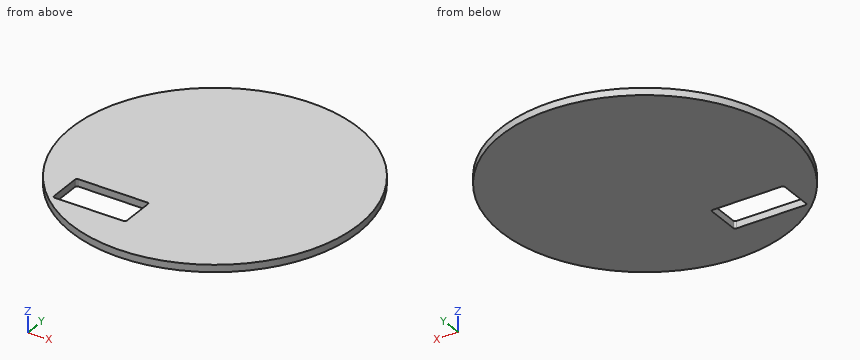
Autodesk Inventor part; units mm, degrees
ref_plane "YZ Plane" through (0, 0, 0) normal (1, 0, 0) x (0, 1, 0)
ref_plane "XZ Plane" through (0, 0, 0) normal (0, 1, 0) x (-1, 0, 0)
ref_plane "XY Plane" through (0, 0, 0) normal (0, 0, 1) x (1, 0, 0)
sketch "Эскиз1" plane through (0, 0, 0) normal (0, 0, 1) x (1, 0, 0)
  circle A0 centre (0, 0) radius 80
  line L0 (-52.7593, -38.063) -> (-52.778, -56.063)
  line L1 (-14.2583, -37.1029) -> (-50.7583, -37.0651)
  line L2 (-12.278, -56.105) -> (-12.2594, -38.105)
  line L3 (-50.779, -57.0651) -> (-14.279, -57.1029)
  line L4 (-51.7583, -37.063) -> (-13.279, -37.063)
  line L5 (-12.279, -38.063) -> (-12.279, -56.105)
  line L6 (-13.279, -57.105) -> (-51.7583, -57.105)
  line L7 (-52.7583, -56.105) -> (-52.7583, -38.063)
  arc A1 (-52.7583, -56.105) -> (-51.7583, -57.105) centre (-51.7583, -56.105) ccw
  arc A2 (-51.7583, -37.063) -> (-52.7583, -38.063) centre (-51.7583, -38.063) ccw
  arc A3 (-13.279, -57.105) -> (-12.279, -56.105) centre (-13.279, -56.105) ccw
  arc A4 (-12.279, -38.063) -> (-13.279, -37.063) centre (-13.279, -38.063) ccw
  point P0 (-52.7583, -37.063)
  dimension "d2" = 160
  dimension "d3" = 1
extrude "Выдавливание1" add sketch "Эскиз1" against normal blind 4
properties part number "нижний эллипс головы"
Build history of the part. All positions in model axes, mm. Round coordinates to 2 decimals unless told otherwise and drop trailing zeros. Loops run counter-clockwise (first coordinate to the right, second up) from the corner with the lowest first, then second, coordinate; pieces in that order, holes last.
Item 1: Saw through at D-D (x = 48). List the corners of the cut face in (y, z), then the cut area to 3 significant figures.
Item 2: Pin check, flat tips, straight feed: P1, Ø2, axis at x = -33.5, z = -2.5, coming from the +Y side; P2, Ø2, axis at y = -51, z = -1.5, coming from the +X side; P3, Ø2, axis at y = -43, z = -1, coming from the -X side. Stop position of each tip, or through.
Item 3: Saw through at A-A (z = -0.85). List the corners of the cut face in (x, y) (3 decimals).
Item 4: Saw through at C-C (y = 14). List the corners of the cut face in (x, z).
Item 5: Saw through at B-B (x = -16.5). List the corners of the cut face in (y, z) (3 decimals).
Item 6: Drill centre lines: line 1 along Y through (x, z) = (-51, -3.55) (3 decimals); line 2 along Y through (x, z) = (-38, -0.55) (3 decimals); line 3 along X through (y, z) = (1.5, -2.7). Where is each one in solid material? Low to high.
Worked answers:
1. outline: (-64, -4) - (64, -4) - (64, 0) - (-64, 0) - close
1. area: 512 mm2
2. P1: stops at y = 73.1
2. P2: stops at x = 62.45
2. P3: stops at x = -68.09
3. outline: circle Ø160 at (0, 0); hole (-52.759, -38.063) - (-52.758, -56.105) arc R1 ccw to (-51.758, -57.105) - (-13.279, -57.105) arc R1.002 ccw to (-12.278, -56.105) - (-12.279, -38.063) arc R1 ccw to (-13.279, -37.063) - (-51.758, -37.063) arc R1.002 ccw to start
4. outline: (-78.77, -4) - (78.77, -4) - (78.77, 0) - (-78.77, 0) - close
5. outline: (-78.28, -4) - (-57.105, -4) - (-57.105, 0) - (-78.28, 0) - close; (-37.063, -4) - (78.28, -4) - (78.28, 0) - (-37.063, 0) - close
6. line 1: y = -61.636 to -57.105, -37.063 to 61.636
6. line 2: y = -70.399 to -57.105, -37.063 to 70.399
6. line 3: x = -79.99 to 79.99
